Geometry: see drawing. Coordinates: mm, zero at the bounding-box minimum. A direction names the side the tool comes from. Give positions to 0.01 mm unless a question says otherwise; leave off trailing zeros. Answer as a JSON object with one key per item and string values. Group by question number.
1. Set-up query: the marked faces 4 and 5. Return all of +Z, -Z, +X, -X, +Y, -Y with unobstructed straight access to the full face (end or side cutting, diameter ignored); none if empty.
2. Material intervals for L1, parallel to Z at x = 73, y = 14 (1 decimal); L2, parallel to Z at x = 99, y = 9.5 (1 decimal); L3, parallel to Z at x = 90, y = 9.5 (1 decimal), sorted ascending. Write a range as [from, to].
3. Pin query (flat end, axial travel): P1, Ø12, axis at x = 124.5, z = 86.5, coming from the -Y side; P2, Ø15.5, axis at x = 125, z = 40.74, coming from the +Y side; P3, Ø2, axis at y = 10.5, z = 48, coming from the +X side; P4, Ø1.5, axis at y = 19.5, z = 132.5, coming from the -X side. Return the tip coordinate at first contact, or that it passes through.
4. Pull-direction query (Z, two-part tool) for the marked faces 1, 2 and 3; classes: +Z half, -Z half, draft (parallel to the pull), parting line (faces both ways), or undercut.
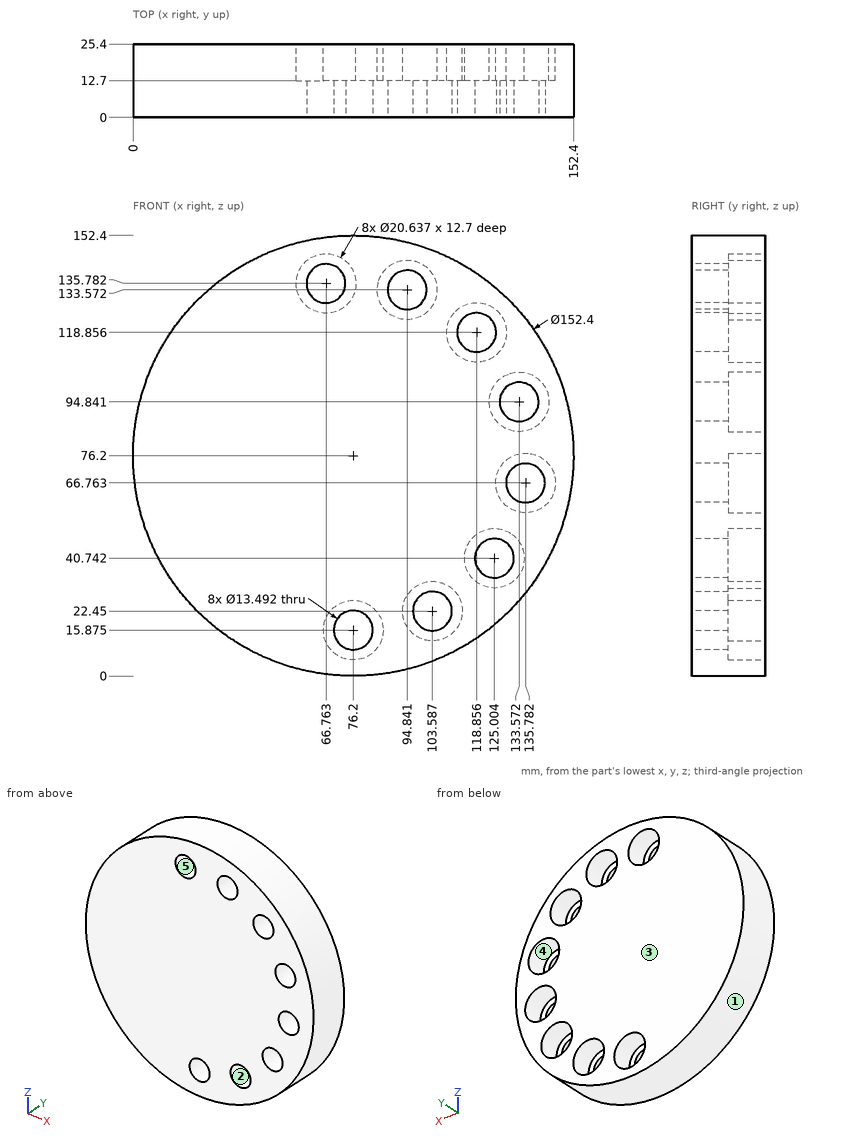
Answer sheet:
{
 "1": {"face 4": "+Y", "face 5": "+Y, -Y"},
 "2": {"L1": "[0.1, 6.1], [25.7, 127.6], [144, 152.3]", "L2": "[3.5, 17.5], [27.4, 128.3], [138.9, 148.9]", "L3": "[1.3, 128.9], [138.3, 151.1]"},
 "3": {"P1": "y = 0", "P2": "y = 12.7", "P3": "x = 147.38", "P4": "x = 24.04"},
 "4": {"face 1": "parting line", "face 2": "undercut", "face 3": "draft"}
}
